Could you check a few things on this model? Use its own coordinates, in mm. Face numbers are marked on the shaded views. A direction names the side the tool comes from. Round coordinates to 2 decimals unless told otherwise and drop trailing zeros. Loops run counter-clockwise (first coordinate to the right, second up) from the corner with the lowest first, then second, coordinate; pieces in that order, holes last. Notation, with made-up numbers: M 28,2.25 L 58,2.25 A21 ccw 58,8.25 Z; hole C -7.75,50.5 d6. An arc over 180 degrees is marked long. Answer in a Markdown table with one row per item.
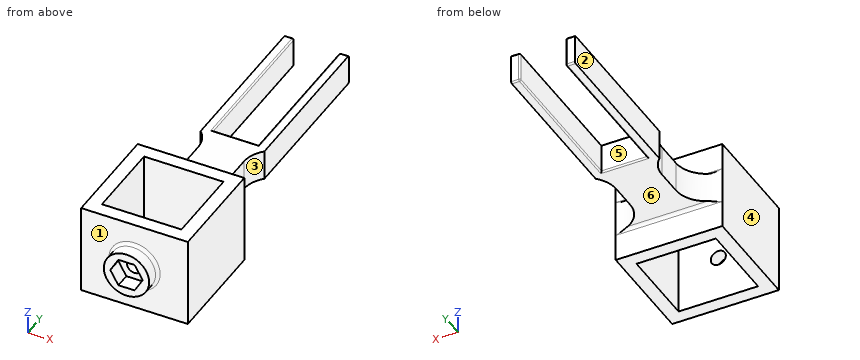
```python
from build123d import *

# Parameters (mm, degrees)
SKETCH2_W               = 25.3
SKETCH2_H               = 25.3
BOSS_EXTRUDE1_DEPTH     = 15
CUT_EXTRUDE1_DEPTH      = 94.422320673
CUT_EXTRUDE1_DEPTH_BACK = 94.422320673
SKETCH3_W               = 10
SKETCH3_H               = 61.95
FILLET1_R               = 10
FILLET2_R               = 1
SKETCH4_R               = 7.5
BOSS_EXTRUDE2_DEPTH     = 5
FILLET3_R               = 1
CUT_EXTRUDE2_REACH      = 101.97
SKETCH5_R               = 2.5
BOSS_EXTRUDE3_DEPTH     = 10
FILLET4_R               = 10
SKETCH11_W              = 15.1
SKETCH11_H              = 10
CUT_EXTRUDE4_DEPTH      = 34.025
FILLET5_R               = 0.5
FILLET6_R               = 0.5
CUT_EXTRUDE5_DEPTH      = 100.956052843
CUT_EXTRUDE5_DEPTH_BACK = 100.956052843
SKETCH12_W              = 26.3
SKETCH12_H              = 26.3


with BuildPart() as part:
    # Sketch2 → Boss-Extrude1 (new, symmetric)
    with BuildSketch(Plane.XY):
        Polygon((-7.55, -53.4), (-7.55, 8.55), (7.55, 8.55), (7.55, -53.4), (17.65, -53.4), (17.65, -88.7), (-17.65, -88.7), (-17.65, -53.4), align=None)
        with Locations((0, -71.05)):
            Rectangle(SKETCH2_W, SKETCH2_H, mode=Mode.SUBTRACT)
    extrude(amount=BOSS_EXTRUDE1_DEPTH, both=True)

    # Sketch3 → Cut-Extrude1 (cut, two sides: drawn at the far end of the back side and taken through both)
    with BuildSketch(Plane(origin=(7.55, 0, 0), x_dir=(0, 0, -1), z_dir=(1, 0, 0)).offset(-CUT_EXTRUDE1_DEPTH_BACK)):
        with Locations((-10, -22.425)):
            Rectangle(SKETCH3_W, SKETCH3_H)
        with Locations((10, -22.425)):
            Rectangle(SKETCH3_W, SKETCH3_H)
    extrude(amount=CUT_EXTRUDE1_DEPTH + CUT_EXTRUDE1_DEPTH_BACK, mode=Mode.SUBTRACT)

    # Fillet1
    fillet1_edges = [part.edges().sort_by_distance(p)[0] for p in [
        (-7.55, -53.4, 0),
        (7.55, -53.4, 0),
    ]]
    fillet(fillet1_edges, radius=FILLET1_R)

    # Fillet2
    fillet2_edges = [part.edges().sort_by_distance(p)[0] for p in [
        (0, -53.4, 5),
        (0, -53.4, -5),
    ]]
    fillet(fillet2_edges, radius=FILLET2_R)

    # Sketch4 → Boss-Extrude2 (add)
    with BuildSketch(Plane.XZ.offset(88.7)):
        Circle(SKETCH4_R)
        Polygon((5.369357503, 0), (2.684678752, 4.65), (-2.684678752, 4.65), (-5.369357503, 0), (-2.684678752, -4.65), (2.684678752, -4.65), align=None, mode=Mode.SUBTRACT)
    extrude(amount=BOSS_EXTRUDE2_DEPTH)

    # Fillet3
    fillet3_edges = [part.edges().sort_by_distance(p)[0] for p in [
        (-7.5, -88.7, 0),
    ]]
    fillet(fillet3_edges, radius=FILLET3_R)

    # Sketch5 → Cut-Extrude2 (cut, up to next)
    with BuildSketch(Plane.XZ.offset(88.7), mode=Mode.PRIVATE) as cut_extrude2_sk1:
        Circle(SKETCH5_R)
    cut_extrude2_tool1 = extrude(cut_extrude2_sk1.sketch, amount=-CUT_EXTRUDE2_REACH, mode=Mode.PRIVATE) & part.part
    add(cut_extrude2_tool1.solids().sort_by_distance((0, -88.7, 0))[0], mode=Mode.SUBTRACT)

    # Sketch9 → Boss-Extrude3 (add)
    with BuildSketch(Plane.XY.offset(5)):
        Polygon((-10.55, -27.475), (-7.55, -27.475), (-7.55, -25.475), (-7.55, 8.55), (-7.55, 25.325), (-10.55, 25.325), (-10.55, -25.325), align=None)
        Polygon((10.55, 25.325), (7.55, 25.325), (7.55, 8.55), (7.55, -25.475), (7.55, -27.475), (10.55, -27.475), (10.55, -25.325), align=None)
        Polygon((7.55, -27.475), (7.55, -25.475), (7.4, -25.475), (-7.4, -25.475), (-7.55, -25.475), (-7.55, -27.475), align=None)
    extrude(amount=-BOSS_EXTRUDE3_DEPTH)

    # Fillet4
    # the kernel refuses this fillet: 10 mm, written as the material it adds along each edge
    with BuildSketch(Plane(origin=(-7.55, -27.475, 5), x_dir=(0, -1, 0), z_dir=(0, 0, -1)), Plane(origin=(7.55, -27.475, -5), x_dir=(0, -1, 0), z_dir=(0, 0, 1))) as fillet4_piece_1:
        with BuildLine():
            CenterArc((7.141428429, 10), FILLET4_R, 224.427004001, 45.572995999)
            Line((0, 3), (-0.142828569, 2.86))
            ThreePointArc((-0.142828569, 2.86), (-0.2, 1.5), (-0.2, 0))
            Line((-0.2, 0), (0, -0.2))
            Line((0, -0.2), (7.141428429, -0.2))
            Line((7.141428429, -0.2), (7.141428429, 0))
        make_face()
    extrude(amount=10)

    # Sketch11 → Cut-Extrude4 (cut)
    with BuildSketch(Plane(origin=(0, 8.55, 0), x_dir=(1, 0, 0), z_dir=(0, 1, 0))):
        Rectangle(SKETCH11_W, SKETCH11_H)
    extrude(amount=-CUT_EXTRUDE4_DEPTH, mode=Mode.SUBTRACT)

    # Fillet5
    fillet5_edges = [part.edges().sort_by_distance(p)[0] for p in [
        (7.55, -0.075, 5),
        (7.55, -0.075, -5),
        (-7.55, -0.075, 5),
        (-7.55, -0.075, -5),
        (0, -25.475, -5),
        (0, -25.475, 5),
    ]]
    fillet(fillet5_edges, radius=FILLET5_R)

    # Fillet6
    fillet6_edges = [part.edges().sort_by_distance(p)[0] for p in [
        (9.3, 25.325, 5),
        (-9.3, 25.325, -5),
        (9.3, 25.325, -5),
        (7.55, 25.325, 0),
        (7.696446609, 25.325, 4.853553391),
        (7.696446609, 25.325, -4.853553391),
        (-7.55, 25.325, 0),
        (-9.3, 25.325, 5),
        (-7.696446609, 25.325, 4.853553391),
        (-7.696446609, 25.325, -4.853553391),
    ]]
    fillet(fillet6_edges, radius=FILLET6_R)

    # Sketch12 → Cut-Extrude5 (cut, two sides: drawn at the far end of the back side and taken through both)
    with BuildSketch(Plane.XY.offset(15).offset(-CUT_EXTRUDE5_DEPTH_BACK)):
        with Locations((0, -71.05)):
            Rectangle(SKETCH12_W, SKETCH12_H)
    extrude(amount=CUT_EXTRUDE5_DEPTH + CUT_EXTRUDE5_DEPTH_BACK, mode=Mode.SUBTRACT)


solid = part.part
```
1) I want a section at A-A, the plane x = 0. State how many separate pieces and enclosed holes the cut face has, plus the area to 3 significant figures.
Computed:
| item | result |
|---|---|
| separate pieces | 3 |
| enclosed holes | 0 |
| area | 556 mm² |
2) I want a section at C-C, the plane x = 12. Please give me the cut outline in (y, z).
Computed:
| item | result |
|---|---|
| outline | M -88.7,-15 L -84.2,-15 L -84.2,15 L -88.7,15 Z; M -57.9,-15 L -53.4,-15 L -53.4,-6 A1 cw -52.4,-5 L -51.72,-5 L -51.72,5 L -52.4,5 A1 cw -53.4,6 L -53.4,15 L -57.9,15 Z |
3) Which directions (+Z, -Z, +X, -X, +Y, -Y) give clear straight access to the entire face, cutting with the end or side of a thin tool? Please do the marked faces 1, 2 and 3.
Computed:
| item | result |
|---|---|
| face 1 | -Y |
| face 2 | +Z, -Z, -X, +Y |
| face 3 | +Z, -Z, +X |
4) I need wall thicknesses on line 1 (X direction, y = -84, z = -5.75); line 2 (Y direction, x = 8.5, z = -9); line 3 (Z direction, x = 0, y = -86). Which ranges of each line are inside material? Lowest first, please.
Computed:
| item | result |
|---|---|
| line 1 | x = -17.65 to -13.15, 13.15 to 17.65 |
| line 2 | y = -88.7 to -84.2, -57.9 to -53.4 |
| line 3 | z = -15 to -2.5, 2.5 to 15 |
5) I want a section at B-B, the plane y = -20.5. Please give me the cut outline in (x, z).
Computed:
| item | result |
|---|---|
| outline | M -10.55,-5 L -8.05,-5 A0.5 ccw -7.55,-4.5 L -7.55,4.5 A0.5 ccw -8.05,5 L -10.55,5 Z; M 7.55,-4.5 A0.5 ccw 8.05,-5 L 10.55,-5 L 10.55,5 L 8.05,5 A0.5 ccw 7.55,4.5 Z |
6) Will these pins go through, and if not, where does the flat tip stop? P1, Ø7, axis at y = -39.5, z = -0.5, coming from the -X side; P2, Ø1.5, axis at y = 3, z = 0.5, coming from the +X side; P3, Ø3, axis at x = -10.5, y = -13.5, coming from the +Z side.
Computed:
| item | result |
|---|---|
| P1 | stops at x = -7.55 |
| P2 | stops at x = 10.55 |
| P3 | stops at z = 5 |
7) I want a section at D-D, the plane y = -38. Please give me the cut outline in (x, z), plus the area to 3 significant figures.
Computed:
| item | result |
|---|---|
| outline | M -7.55,-5 L 7.55,-5 L 7.55,5 L -7.55,5 Z |
| area | 151 mm² |
8) If we mould it in two halves opening along X, with no side actions, what happens to the marked faces 4, 5 and 6? For each: released by +X, released by -X, zero draft, split by the parting line, or undercut.
Computed:
| item | result |
|---|---|
| face 4 | released by -X |
| face 5 | undercut |
| face 6 | zero draft |
